Autodesk Inventor part; units mm, degrees
ref_plane "YZ Plane" through (0, 0, 0) normal (1, 0, 0) x (0, 1, 0)
ref_plane "XZ Plane" through (0, 0, 0) normal (0, 1, 0) x (-1, 0, 0)
ref_plane "XY Plane" through (0, 0, 0) normal (0, 0, 1) x (1, 0, 0)
sketch "スケッチ1" plane through (0, 0, 0) normal (0, 0, 1) x (1, 0, 0)
  line L0 (-5, -15) -> (5, -15)
  line L1 (5, -15) -> (5, 15)
  line L2 (5, 15) -> (-5, 15)
  line L3 (-5, 15) -> (-5, -15)
  line L4 (-5, -15) -> (5, 15) construction
  line L5 (5, -15) -> (-5, 15) construction
  point P0 (0, 0)
  dimension "d0" = 10
  dimension "d1" = 30
extrude "押し出し1" add sketch "スケッチ1" along normal mid plane 90
sketch "スケッチ2" plane through (0, 0, 45) normal (0, 0, 1) x (1, 0, 0)
  line L0 (5, 15) -> (-5, 15)
  line L1 (5, -15) -> (5, 15)
  line L2 (-5, -15) -> (5, -15)
  point P0 (0, 0)
  point P1 (0, 10)
  point P2 (0, -10)
  dimension "d4" = 5
  dimension "d5" = 5
  dimension "d6" = 5
  dimension "d7" = 5
hole "穴1" at (0, 10, 45) at (0, -10, 45) direction (0, 0, -1) diameter 2.5 depth 10 tip angle 118
sketch "スケッチ3" plane through (0, 0, -45) normal (0, 0, -1) x (-1, 0, 0)
  circle A0 centre (0, 10) radius 1.25
  circle A1 centre (0, -10) radius 1.25
  point P0 (0, 0)
hole "穴2" at (0, 10, -45) at (0, -10, -45) direction (0, 0, 1) diameter 2.5 depth 10 tip angle 118
sketch "スケッチ4" plane through (5, -15, 45) normal (1, 0, 0) x (0, 0, -1)
  line L0 (90, 30) -> (0, 30)
  line L1 (0, 0) -> (0, 30)
  point P0 (45, 15)
  point P1 (45, 25)
  point P2 (45, 5)
  point P3 (45, 30)
  dimension "d22" = 5
  dimension "d23" = 20
  dimension "d24" = 45
  dimension "d25" = 45
hole "穴3" at (5, 10, 0) at (5, -10, 0) direction (-1, 0, 0) diameter 4.5 end through all
properties part number "ベースパーツ_実験装置取り付け部分"
Geometry: final body of the model. Coordinates: model frame, mm. A direction names the side the tool comes from. Round coordinates to 2 decimals unless told otherwise and drop trailing zeros. Write each loop counter-clockwise with the first axis right and the second up, starting at its lowest first coordinate (ties: lowest second). Pieces come first, ordered by that corner, then holes. Notation, with made-up numbers: (-7.75, 30) -> (47.25, 30) arc R10 ccw to (47.25, 42) -> close; hole circle Ø5 at (-27.5, -17). An arc over 180 degrees is marked (long way). Return JSON: item names as keys, results as strings.
Q1. Section A-A on z = 0. Return the cut outline in (x, y), and give its area (3 significant figures).
From the geometry:
{"outline": "(-5, -15) -> (5, -15) -> (5, -12.25) -> (-5, -12.25) -> close; (-5, -7.75) -> (5, -7.75) -> (5, 7.75) -> (-5, 7.75) -> close; (-5, 12.25) -> (5, 12.25) -> (5, 15) -> (-5, 15) -> close", "area": "210 mm2"}
Q2. First-contact query: pin 1 Ø7 at (y, z) = (-10, 0) entering from +X; pin 2 Ø1.5 at (x, y) = (0, 10) entering from +Z; pin 3 Ø2 at (x, y) = (0, -10) entering from -Z; pin 4 Ø3.5 at (y, z) = (10, 0) entering from +X. Flat tips, straight axial feed; report the tip coordinate or a pass-through.
From the geometry:
{"pin 1": "x = 5", "pin 2": "z = 34.7", "pin 3": "z = -34.85", "pin 4": "through"}
Q3. Section B-B on z = -37.5. Return the cut outline in (x, y), and give its area (3 significant figures).
From the geometry:
{"outline": "(-5, -15) -> (5, -15) -> (5, 15) -> (-5, 15) -> close; hole circle Ø2.5 at (0, -10); hole circle Ø2.5 at (0, 10)", "area": "290 mm2"}
Q4. Ray query, line 1 (Y direction, x = 0, z = -42); line 2 (Y direction, x = 2.5, z = 0); line 3 (X direction, y = 10, z = 39.25). Return the intervals inside material, ascending.
From the geometry:
{"line 1": "-15 to -11.25, -8.75 to 8.75, 11.25 to 15", "line 2": "-15 to -12.25, -7.75 to 7.75, 12.25 to 15", "line 3": "-5 to -1.25, 1.25 to 5"}
Q5. Mould query, pull axis Z, two halves, no side actions, for faces 4 (the cylindrical face through (-0.05, 8.75, -39.93)), 5 (the cylindrical face through (-0.07, -11.897, -1.21)), 6 (the flat face through (0, 0, -45)). Classes: +Z half, -Z half, draft (parallel to the pull), parting line (faces both ways), or undercut.
From the geometry:
{"face 4": "draft", "face 5": "undercut", "face 6": "-Z half"}
Q6. Set-up query: faces 1 (the cylindrical face through (-0.07, 7.77, 0.29)), 2 (the cylindrical face through (-0.05, -8.75, 39.93)), 3 (the cylindrical face through (-0.05, -11.25, -39.93)). Return all of +Z, -Z, +X, -X, +Y, -Y with unobstructed straight access to the full face (end or side cutting, diameter ignored); none if empty.
From the geometry:
{"face 1": "+X, -X", "face 2": "+Z", "face 3": "-Z"}
